Check sheet for the drawn part. Datum: minimum x, y, z corner. Units: mm. A direction names the side the tool comes from. Coordinates: 2 decimals unless noted, no trailing zeros. Loops run counter-clockwise (first coordinate to the right, second up) from the corner with the lowest first, then second, coordinate; pieces in that order, holes last. Notation, with made-up numbers: (65.25, 83) - (94.25, 83) arc R25 cw to (94.25, 103) - close; hole circle Ø4 at (-2.5, 43). An arc over 180 degrees is marked (long way). Write item = value, one per line. Start each with the question number.
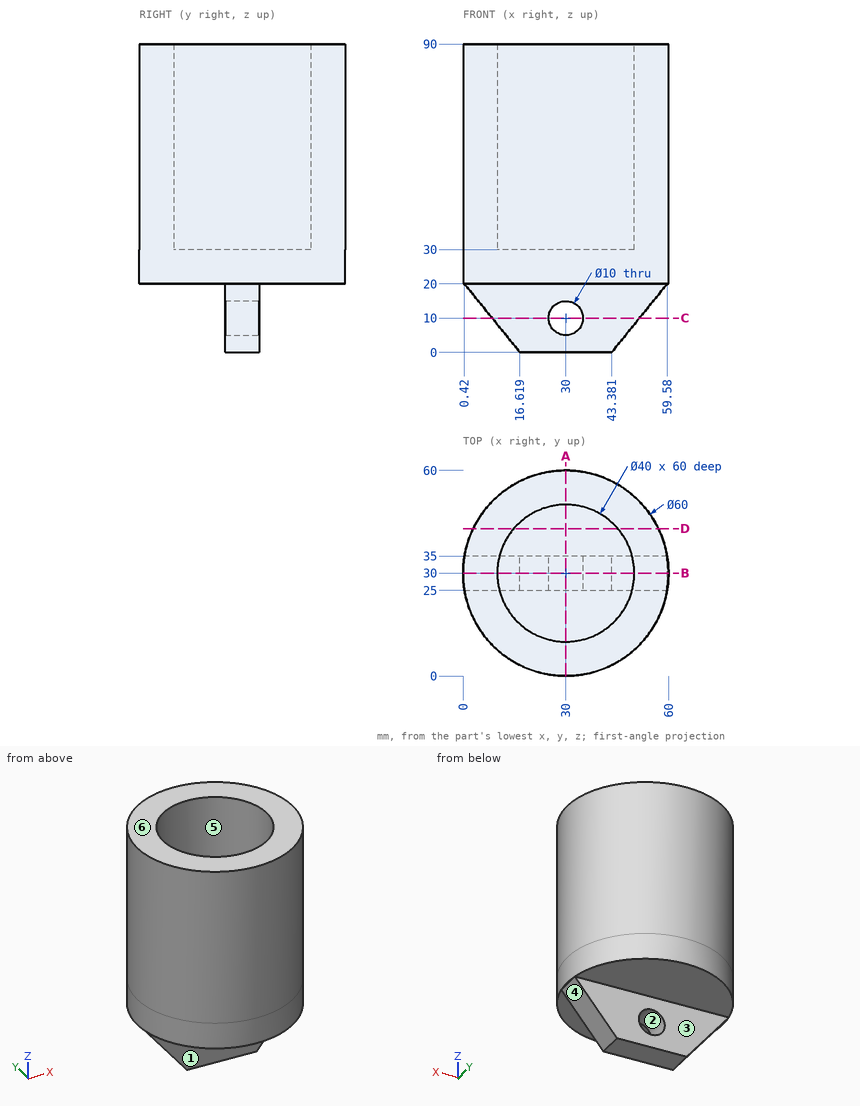
(1) Sectioned sample at A-A on x = 30. Enter the section's corners in (y, z), plus the area to 3 significant figures.
(2) Tool access check on the marked faces 1, 2 and 3. Record the directions out of +Z, -Z, +X, -X, +Y, -Y that give a thin tool (end or side, any length) a straight path to the whole face; none if there is none.
(3) Depth check by flat-ended pin: pin 1 (8 mm diameter, centred on x = 35, z = 74, fed in from +Y); pin 2 (10 mm diameter, centred on x = 46.5, z = 27, fed in from -Y); pin 3 (6 mm diameter, centred on y = 39.5, z = 34.5, fed in from +X). Enter the tip coordinate at first touch or a pass-through.
(4) Draft check along X on the marked faces 4, 5 and 6. Enter one of: pulls with the +X half, pulls with the -X half, needs draft (parallel to the pull), parting line crosses it, or undercut.
(5) Scan lines: line 1 (Z direction, x = 30, y = 29.25); line 2 (X direction, y = 30.5, z = 72.5) (1 decimal); line 3 (Y direction, x = 33, z = 52). Record each from-to range of solid material in increasing order.
(6) Sectioned sample at D-D on y = 43. Enter the section's corners in (x, z), plus the area to 3 significant figures.
(7) Sectioned sample at B-B on y = 30. Enter the section's corners in (x, z), plus the area to 3 significant figures.
(8) Sectioned sample at C-C on z = 10. Enter the section's corners in (x, y), plus the area to 3 significant figures.
Working result:
q1.outline = (0, 20) - (25, 20) - (25, 15) - (35, 15) - (35, 20) - (60, 20) - (60, 90) - (50, 90) - (50, 30) - (10, 30) - (10, 90) - (0, 90) - close; (25, 0) - (35, 0) - (35, 5) - (25, 5) - close
q1.area = 1,900 mm2
q2.face_1 = -Z, +X, -X, -Y
q2.face_2 = +Y, -Y
q2.face_3 = -Z, +X, -X, +Y
q3.pin_1 = 59.98
q3.pin_2 = 2.29
q3.pin_3 = 59.29
q4.face_4 = pulls with the +X half
q4.face_5 = undercut
q4.face_6 = needs draft
q5.line_1 = 0 to 5, 15 to 30
q5.line_2 = 0 to 10, 50 to 60
q5.line_3 = 0.15 to 10.23, 49.77 to 59.85
q6.outline = (2.96, 20) - (57.04, 20) - (57.04, 90) - (45.2, 90) - (45.2, 30) - (14.8, 30) - (14.8, 90) - (2.96, 90) - close
q6.area = 1,960 mm2
q7.outline = (0, 20) - (0.42, 20) - (16.62, 0) - (43.38, 0) - (59.58, 20) - (60, 20) - (60, 90) - (50, 90) - (50, 30) - (10, 30) - (10, 90) - (0, 90) - close; hole circle Ø10 at (30, 10)
q7.area = 2,580 mm2
q8.outline = (8.52, 25) - (25, 25) - (25, 35) - (8.52, 35) - close; (35, 25) - (51.48, 25) - (51.48, 35) - (35, 35) - close
q8.area = 330 mm2
